Can you work these out from the model? Positions are in its coordinate system, mm. A direction names the side the tool comes from. Coordinates: 2 decimals unless noted, no trailing zeros. Order: outer loops, then holes, each group sorted by start corner. A loop starts at its lowest first (then second) coordinate and runs counter-clockwise, first axis right, second up. Notation, with made-up numbers: (57.25, -2.5) -> (105.25, -2.5) arc R25 cw to (105.25, 13.5) -> close; hole circle Ø11 at (88, 83). An arc over 180 degrees is marked (long way). Return JSON: item names as keys, results as strings. Group by question number.
1) If we section it at B-B, the plane z = 0: Please give me the cut outline in (x, y).
2) For faces 4 (the flat face through (2, 14.5, -10)), 5 (the flat face through (2, 20.175, -17)), 6 (the flat face through (5, 2, 5)), 7 (the flat face through (2, 9, 21)), 8 (the flat face through (-2, -15, -5)), which set-ups out of +Z, -Z, +X, -X, +Y, -Y let a thin tool reach every point of the face, with its end or its side?
3) If I drill on probe 1 along Y at (x, z) = (2.5, -8) (3 decimals); probe 2 along Y at (x, z) = (1.3, 0); probe 3 along Y at (x, z) = (3.25, 22.5), over which ranges is the centre line in solid material (lowest first)? Write a range as from..to.
4) If we section it at A-A, the plane y = 0: State how many separate pieces and enclosed holes the cut face has, then the cut area to 3 significant figures.
5) Thinking about a two-plate mould opening in Y: for faces 1 (the flat face through (2, 19, -15.5)), 2 (the flat face through (2, 17, 24)), 3 (the cylindrical face through (3.48, 0.07, -9.6)), which applies, +Y half, -Y half, draft (parallel to the pull), parting line (faces both ways), or undercut?
6) For pin 1 (1.6 mm diameter, centred on x = 1.5, y = 19, fed in from -Z); pin 2 (6 mm diameter, centred on y = 10, z = 1, fed in from -X); pin 3 (3.5 mm diameter, centred on x = 3, y = 19, fed in from +Z), each with a flat end and sliding along its axis, tell me the tip position at first contact or that it passes through.
7) If we section it at C-C, the plane x = -0.75: Please give me the cut outline in (y, z).
8) If we section it at D-D, the plane z = 21.2: Please give me the cut outline in (x, y), then the cut area to 3 significant figures.
from build123d import *

# Parameters (mm, degrees)
BOSS_EXTRUDE1_DEPTH = 5
SKETCH2_R           = 13.95
CUT_EXTRUDE1_DEPTH  = 2
SKETCH3_R           = 4.9
CUT_EXTRUDE2_DEPTH  = 3.9624
CUT_EXTRUDE3_REACH  = 37.618
SKETCH4_R           = 1.6
SKETCH4_R_2         = 5.1
SKETCH5_R           = 2
CUT_EXTRUDE4_DEPTH  = 36.712340147
FILLET1_R           = 10
BOSS_EXTRUDE2_START = 4
BOSS_EXTRUDE2_DEPTH = 4
FILLET2_R           = 1
CHAMFER1_SIZE       = 0.2
SKETCH7_R           = 0.15
SKETCH10_R          = 0.15


with BuildPart() as part:
    # Sketch1 → Boss-Extrude1 (new body)
    with BuildSketch(Plane(origin=(0, 0, 0), x_dir=(0, 0, -1), z_dir=(1, 0, 0))):
        Polygon((-29.2, 17), (-29.2, -17), (20, -17), (20, 17), (18, 17), (18, 20.175), (15.5, 20.175), (15.5, 17), (13.15, 17), (13.15, 14.5), (14.15, 14.5), (14.15, 12.5), (13.15, 12.5), (13.15, 9), (10.85, 9), (10.85, 12.5), (9.85, 12.5), (9.85, 14.5), (10.85, 14.5), (10.85, 17), (8.5, 17), (8.5, 20.175), (6, 20.175), (6, 17), (-15.2, 17), (-15.2, 20.175), (-17.7, 20.175), (-17.7, 17), (-20.05, 17), (-20.05, 14.5), (-19.05, 14.5), (-19.05, 12.5), (-20.05, 12.5), (-20.05, 9), (-22.35, 9), (-22.35, 12.5), (-23.35, 12.5), (-23.35, 14.5), (-22.35, 14.5), (-22.35, 17), (-24.7, 17), (-24.7, 20.175), (-27.2, 20.175), (-27.2, 17), align=None)
    extrude(amount=BOSS_EXTRUDE1_DEPTH)

    # Sketch2 → Cut-Extrude1 (cut)
    with BuildSketch(Plane.ZY):
        Circle(SKETCH2_R)
    extrude(amount=-CUT_EXTRUDE1_DEPTH, mode=Mode.SUBTRACT)

    # Sketch3 → Cut-Extrude2 (cut)
    with BuildSketch(Plane(origin=(5, 0, 0), x_dir=(0, 0, -1), z_dir=(1, 0, 0))):
        with Locations((-21.2, 0)):
            Circle(SKETCH3_R)
    extrude(amount=-CUT_EXTRUDE2_DEPTH, mode=Mode.SUBTRACT)

    # Sketch4 → Cut-Extrude3 (cut, up to next)
    with BuildSketch(Plane.ZY.offset(-2), mode=Mode.PRIVATE) as cut_extrude3_sk1:
        with Locations((-8, 0)):
            Circle(SKETCH4_R)
    cut_extrude3_tool1 = extrude(cut_extrude3_sk1.sketch, amount=-CUT_EXTRUDE3_REACH, mode=Mode.PRIVATE) & part.part
    # Sketch4 → Cut-Extrude3 (cut, up to next)
    with BuildSketch(Plane.ZY.offset(-2), mode=Mode.PRIVATE) as cut_extrude3_sk2:
        with Locations((8, 0)):
            Circle(SKETCH4_R)
    cut_extrude3_tool2 = extrude(cut_extrude3_sk2.sketch, amount=-CUT_EXTRUDE3_REACH, mode=Mode.PRIVATE) & part.part
    # Sketch4 → Cut-Extrude3 (cut, up to next)
    with BuildSketch(Plane.ZY.offset(-2), mode=Mode.PRIVATE) as cut_extrude3_sk3:
        Circle(SKETCH4_R_2)
    cut_extrude3_tool3 = extrude(cut_extrude3_sk3.sketch, amount=-CUT_EXTRUDE3_REACH, mode=Mode.PRIVATE) & part.part
    add(cut_extrude3_tool1.solids().sort_by_distance((2, 0, -8))[0], mode=Mode.SUBTRACT)
    add(cut_extrude3_tool2.solids().sort_by_distance((2, 0, 8))[0], mode=Mode.SUBTRACT)
    add(cut_extrude3_tool3.solids().sort_by_distance((2, 0, 0))[0], mode=Mode.SUBTRACT)

    # Sketch5 → Cut-Extrude4 (cut, through all)
    with BuildSketch(Plane(origin=(1.0376, 0, 0), x_dir=(0, 0, -1), z_dir=(1, 0, 0))):
        with Locations((-21.2, 0)):
            Circle(SKETCH5_R)
    extrude(amount=-CUT_EXTRUDE4_DEPTH, mode=Mode.SUBTRACT)

    # Fillet1
    fillet1_edges = [part.edges().sort_by_distance(p)[0] for p in [
        (2.5, -17, -20),
        (2.5, -17, 29.2),
    ]]
    fillet(fillet1_edges, radius=FILLET1_R)

    # Sketch6 → Boss-Extrude2 (add)
    with BuildSketch(Plane.ZY.offset(BOSS_EXTRUDE2_START)):
        with BuildLine():
            Line((-5, -13.02315246), (-5, -17))
            Line((-5, -17), (5, -17))
            Line((5, -17), (5, -13.02315246))
            ThreePointArc((5, -13.02315246), (0, -13.95), (-5, -13.02315246))
        make_face()
    extrude(amount=-BOSS_EXTRUDE2_DEPTH)

    # Fillet2
    fillet2_edges = [part.edges().sort_by_distance(p)[0] for p in [
        (-2, -13.02315246, 5),
        (-2, -13.02315246, -5),
        (-2, -17, -5),
        (-2, -17, 5),
        (-4, -17, 0),
    ]]
    fillet(fillet2_edges, radius=FILLET2_R)

    # Chamfer1
    chamfer1_edges = [part.edges().sort_by_distance(p)[0] for p in [
        (5, 0, 26.1),
    ]]
    chamfer(chamfer1_edges, length=CHAMFER1_SIZE)

    # Sketch7 → Cut-Revolve1 (revolve, cut)
    with BuildSketch(Plane(origin=(0, 0, 0), x_dir=(1, 0, 0), z_dir=(0, 1, 0)), mode=Mode.PRIVATE) as cut_revolve1_sk:
        with Locations((1.9, -13.85)):
            Circle(SKETCH7_R)
    revolve(cut_revolve1_sk.sketch.rotate(Axis((5, 0, 0), (-1, 0, 0)), 285.519036576), axis=Axis((5, 0, 0), (-1, 0, 0)), mode=Mode.SUBTRACT)

    # Sketch10 → Cut-Revolve2 (revolve, cut)
    with BuildSketch(Plane(origin=(0, 0, 0), x_dir=(1, 0, 0), z_dir=(0, 1, 0))):
        with Locations((1.1376, -16.4)):
            Circle(SKETCH10_R)
    revolve(axis=Axis((0, 0, 21.2), (1, 0, 0)), mode=Mode.SUBTRACT)


solid = part.part
Result sheet:
{
 "1": {"outline": "(-4, -16) arc R1 ccw to (-3, -17) -> (5, -17) -> (5, -5.1) -> (2, -5.1) -> (2, -13.74) arc R0.15 cw (long way) to (1.79, -13.95) -> (-4, -13.95) -> close; (0, 13.95) -> (1.79, 13.95) arc R0.15 cw (long way) to (2, 13.74) -> (2, 5.1) -> (5, 5.1) -> (5, 17) -> (0, 17) -> close"},
 "2": {"face 4": "+X, -X", "face 5": "+Z, -Z, +X, -X, +Y", "face 6": "+Z, -Z, +X, +Y, -Y", "face 7": "+X, -X, +Y", "face 8": "-Z, -X, +Y, -Y"},
 "3": {"probe 1": "y = -17..-1.6, 1.6..20.175", "probe 2": "y = -17..-13.95, 13.95..17", "probe 3": "y = -16.44..-4.72, 4.72..12.5, 14.5..17"},
 "4": {"separate pieces": "5", "enclosed holes": "0", "area": "97.3 mm2"},
 "5": {"face 1": "draft", "face 2": "+Y half", "face 3": "undercut"},
 "6": {"pin 1": "stops at z = -18", "pin 2": "stops at x = 2", "pin 3": "stops at z = 27.2"},
 "7": {"outline": "(-17, -4) arc R1 ccw to (-16, -5) -> (-14.4, -5) arc R1 ccw to (-13.44, -3.73) arc R13.95 cw to (-13.44, 3.73) arc R1 ccw to (-14.4, 5) -> (-16, 5) arc R1 ccw to (-17, 4) -> close"},
 "8": {"outline": "(0, -16.8) -> (5, -16.8) -> (5, -5.1) -> (4.8, -4.9) -> (1.25, -4.9) arc R0.15 cw (long way) to (1.04, -4.69) -> (1.04, -2) -> (0, -2) -> close; (0, 2) -> (1.04, 2) -> (1.04, 4.69) arc R0.15 cw (long way) to (1.25, 4.9) -> (4.8, 4.9) -> (5, 5.1) -> (5, 9) -> (0, 9) -> close", "area": "85.9 mm2"}
}
